Check sheet for the modelled part. Datum: model origin and axes. Units: mm. A direction names the side the tool comes from. Round coordinates to 2 decimals unless told otherwise and drop trailing zeros. Order: outer loops, then holes, each group sorted by start corner. A loop starts at its lowest first (then second) coordinate and runs counter-clockwise, first axis right, second up.
Q1. Mould release check, pull along Y, two halves, no side actions. Record for faces 6 (the cylindrical face through (8.06, 10.57, -18.1)), 7 (the cylindrical face through (8.06, -10.6, -18.07)), 8 (the cylindrical face through (7.25, 19.43, -18.1)), 9 (the flat face through (-2, -20, -15)): +Y half, -Y half, draft (parallel to the pull), parting line (faces both ways), or undercut.
Q2. Cross-section at A-A on x = 6.5. Record the cut outline in (y, z) (3 decimals), then the cut area to 3 significant figures.
Q3. Scan lines: probe 1 along Z at (x, y) = (5.75, 0) (3 decimals); probe 2 along X at (y, z) = (-15, -20.35); probe 3 along X at (y, z) = (-7, 15). Record each from-to range of solid material in increasing order.
Q4. Set-up check for faces 1 (the cylindrical face through (7.462, -0.84, 6.283)), 2 (the flat face through (8, 10, -21)), 3 (the flat face through (2, 0, -22.5)), 4 (the cylindrical face through (2.32, 18.5, -8.34)), 5 (the cylindrical face through (11.677, -13.014, -20.035)): record each of +Z, -Z, +X, -X, +Y, -Y from which the full face is reachable in a straight line by a thin tool's end or side.
Q5. Depth check by flat-ended pin: P1, Ø6.5, axis at x = 8.5, y = -16, coming from the +Z side; P2, Ø2, axis at x = 2.5, y = -15, coming from the +Z side; P3, Ø3, axis at x = 8.5, y = -1, coming from the +Z side (3 decimals). Enter the tip coordinate at first touch or a pass-through.
Solid Edge part; units mm, degrees
sketch "Sketch1" plane through (0, 0, 0) normal (0, -1, 0) x (1, 0, 0)
  line L0 (3.75, 22.5) -> (3.75, -22.5)
  line L1 (3.75, -22.5) -> (-3.75, -22.5)
  line L2 (-3.75, -22.5) -> (-3.75, 22.5)
  line L3 (-3.75, 22.5) -> (3.75, 22.5)
extrude "Protrusion1" add sketch "Sketch1" along normal mid plane 40
fillet "Round_1" radius 20 2 edges at (0, -20, 22.5) (0, 20, 22.5)
sketch "Sketch2" plane through (3.75, 0, 0) normal (1, 0, 0) x (0, 1, 0)
  circle A0 centre (0, 2.5) radius 3.875
extrude "ExtrudedProtrusion_2" add sketch "Sketch2" along normal mid plane 15
fillet "Round_2" radius 5 3 edges at (3.75, 0, 22.5) (3.75, -20, -10) (3.75, 20, -10)
fillet "Round_3" radius 1 2 edges at (3.75, 0, 6.375) (11.25, -3.875, 2.5)
sketch "Sketch3" plane through (0, 0, -22.5) normal (0, 0, -1) x (0, 1, 0)
  circle A0 centre (-15, 12.5) radius 2.15
  line L0 (-20, 17.5) -> (-10, 17.5)
  line L1 (-10, 17.5) -> (-10, -3.75)
  line L2 (-10, -3.75) -> (-20, -3.75)
  line L3 (-20, -3.75) -> (-20, 17.5)
extrude "ExtrudedProtrusion_3" add sketch "Sketch3" against normal blind 5
fillet "Round_4" radius 5 2 edges at (17.5, -20, -20) (17.5, -10, -20)
mirror "Mirror1" about plane through (0, 0, 0) normal (0, -1, 0) of "ExtrudedProtrusion_3"
fillet "Round1" radius 5 2 edges at (17.5, 20, -20) (17.5, 10, -20)
sketch "Sketch4" plane through (-3.75, 0, 0) normal (-1, 0, 0) x (0, -1, 0)
  circle A0 centre (0, 2.5) radius 2.05
extrude "Cutout1" cut sketch "Sketch4" against normal through all
fillet "Round_6" radius 2 1 edges at (-3.75, 2.05, 2.5)
fillet "Round_7" radius 2 4 edges at (8.125, -10, -17.5) (5.625, -20, -17.5) (8.125, 10, -17.5) (5.625, 20, -17.5)
Results found:
1. face 6: undercut
1. face 7: undercut
1. face 8: +Y half
1. face 9: -Y half
2. outline: (-20, -22.5) - (-10, -22.5) - (-10, -19.5) arc R2 ccw to (-12, -17.5) - (-18, -17.5) arc R2 ccw to (-20, -19.5) - close; circle Ø7.75 at (0, 2.5); (10, -22.5) - (20, -22.5) - (20, -19.5) arc R2 ccw to (18, -17.5) - (12, -17.5) arc R2 ccw to (10, -19.5) - close; hole circle Ø4.1 at (0, 2.5)
2. area: 131 mm2
3. probe 1: z = -1.375 to 0.45, 4.55 to 6.375
3. probe 2: x = -3.75 to 10.35, 14.65 to 17.5
3. probe 3: x = -3.75 to 3.75
4. face 1: +X
4. face 2: +Z, -Z, +X
4. face 3: -Z, +X, -X, +Y, -Y
4. face 4: +Z, +X, +Y
4. face 5: +Z, -Z
5. P1: stops at z = -17.5
5. P2: stops at z = 14.97
5. P3: stops at z = 6.375
